Geometry: final body of the model. Coordinates: model frame, mm. Face numbers are marked on the shaded views. A direction names the side the tool comes from. Coordinates: 2 decimals unless noted, no trailing zeros. Write each loop counter-clockwise with the first axis right and the second up, starting at its lowest first coordinate (ties: lowest second). Pieces come first, ordered by that corner, then holes. Notation, with made-up numbers: M 43.25,64 L 80.25,64 A20 cw 80.25,74 Z; hole C 39,74.25 d8. An arc over 180 degrees is marked long. Write item = value, one per line. Start each with the question number.
Item 1: First-contact query: pin 1 Ø3.5 at (x, z) = (5.6, -28.87) entering from +Y; pin 2 Ø0.5 at (x, y) = (7, 3.5) entering from +Z; pin 3 Ø1.6 at (y, z) = (1.5, -35.5) entering from +X. Flat tips, straight axial feed; report the tip coordinate or a pass-through.
Item 2: Section A-A on x = 25.25. Output: boundary loops of the cut face in (y, z), plus the area to 3 significant figures.
Item 3: Pull-direction query (Z, two-part tool) for the marked faces 3 and 4; classes: +Z half, -Z half, draft (parallel to the pull), parting line (faces both ways), or undercut.
Item 4: Reachability of the marked faces 1 and 2 from +Z, -Z, +X, -X, +Y, -Y: full face, straight path, thin tool, end or side. Return the list, or none.
Item 5: Ray query, L1, parallel to X at y = 1.7, z = 2.45; L2, parallel to Z at x = 3, y = 0.35; L3, parallel to Z at x = 16.5, y = 2.75. Return the intervals inside material, ascending. Write a range as [from, to].
Item 6: Section B-B on z = -16. Output: boundary loops of the cut face in (x, y).
Item 7: Section C-C on z = -3. Output: boundary loops of the cut face in (x, y).
from build123d import *

# Parameters (mm, degrees)
SKETCH_1_W           = 20
SKETCH_1_H           = 35.74
EXTRUDE_1_DEPTH      = 4
SKETCH_2_W           = 8.8
SKETCH_2_H           = 8.5
SKETCH_2_H_2         = 9.8
EXTRUDE_2_DEPTH      = 4
SKETCH_3_R           = 13.5
CUT_EXTRUDE_1_DEPTH  = 10
SKETCH_4_W           = 9
SKETCH_4_H           = 5
CUT_EXTRUDE_2_DEPTH  = 1
SKETCH_5_W           = 9.228972975
SKETCH_5_H           = 4
EXTRUDE_3_DEPTH      = 10
SKETCH_6_R           = 1.6
CUT_EXTRUDE_3_DEPTH  = 10
SKETCH_7_R           = 1.6
CUT_EXTRUDE_4_DEPTH  = 55.679901244
SKETCH_8_W           = 11.2
SKETCH_8_H           = 4
EXTRUDE_4_DEPTH      = 4
SKETCH_9_R           = 1.65
CUT_EXTRUDE_5_DEPTH  = 55.679901244
SKETCH_10_W          = 10
SKETCH_10_H          = 4
EXTRUDE_5_DEPTH      = 7
SKETCH_11_R          = 1.65
CUT_EXTRUDE_6_DEPTH  = 8
SKETCH_12_W          = 6.6
SKETCH_12_H          = 5
CUT_EXTRUDE_7_DEPTH  = 1
SKETCH_13_R          = 1.55
CUT_EXTRUDE_8_DEPTH  = 5
SKETCH_14_W          = 18.2
SKETCH_14_H          = 1.73
EXTRUDE_6_DEPTH      = 4
SKETCH_16_W          = 10
SKETCH_16_H          = 8
CUT_EXTRUDE_9_DEPTH  = 1
CUT_EXTRUDE_10_DEPTH = 2.4
FILLET_1_R           = 4
CUT_EXTRUDE_11_DEPTH = 55.679901244
CHAMFER_1_SIZE       = 0.4


with BuildPart() as part:
    # 草图1 → 凸台-拉伸1 (new body)
    with BuildSketch(Plane(origin=(0, 0, 0), x_dir=(1, 0, 0), z_dir=(0, 1, 0))):
        with Locations((10, 17.87)):
            Rectangle(SKETCH_1_W, SKETCH_1_H)
    extrude(amount=EXTRUDE_1_DEPTH)

    # 草图2 → 凸台-拉伸2 (add)
    with BuildSketch(Plane.XZ):
        with Locations((15.6, 4.25)):
            Rectangle(SKETCH_2_W, SKETCH_2_H)
        with Locations((15.6, -40.64)):
            Rectangle(SKETCH_2_W, SKETCH_2_H_2)
    extrude(amount=-EXTRUDE_2_DEPTH)

    # 草图3 → 切除-拉伸1 (cut)
    with BuildSketch(Plane(origin=(0, 0, 0), x_dir=(-1, 0, 0), z_dir=(0, -1, 0))):
        with Locations((-24, 21.6)):
            Circle(SKETCH_3_R)
    extrude(amount=-CUT_EXTRUDE_1_DEPTH, mode=Mode.SUBTRACT)

    # 草图4 → 切除-拉伸2 (cut)
    with BuildSketch(Plane(origin=(0, 0, 0), x_dir=(-1, 0, 0), z_dir=(0, -1, 0))):
        with Locations((-13.5, -0.75)):
            Rectangle(SKETCH_4_W, SKETCH_4_H)
    extrude(amount=-CUT_EXTRUDE_2_DEPTH, mode=Mode.SUBTRACT)

    # 草图5 → 凸台-拉伸3 (add)
    with BuildSketch(Plane(origin=(20, 0, 0), x_dir=(0, 0, -1), z_dir=(1, 0, 0))):
        with Locations((-3.885513513, 2)):
            Rectangle(SKETCH_5_W, SKETCH_5_H)
    extrude(amount=EXTRUDE_3_DEPTH)

    # 草图6 → 切除-拉伸3 (cut)
    with BuildSketch(Plane(origin=(0, 0, 0), x_dir=(-1, 0, 0), z_dir=(0, -1, 0))):
        with Locations(Location((-15.2, 36.59, 0), (0, 0, 90))):
            Circle(SKETCH_6_R)
        with Locations(Location((-25.25, -2.45, 0), (0, 0, 90))):
            Circle(SKETCH_6_R)
    extrude(amount=-CUT_EXTRUDE_3_DEPTH, mode=Mode.SUBTRACT)

    # 草图7 → 切除-拉伸4 (cut, through all)
    with BuildSketch(Plane(origin=(0, 0, 0), x_dir=(-1, 0, 0), z_dir=(0, -1, 0))):
        with Locations(Location((-5.6, 28.87, 0), (0, 0, 90))):
            Circle(SKETCH_7_R)
        with Locations(Location((-5.6, 6.87, 0), (0, 0, 90))):
            Circle(SKETCH_7_R)
    extrude(amount=-CUT_EXTRUDE_4_DEPTH, mode=Mode.SUBTRACT)

    # 草图8 → 凸台-拉伸4 (add)
    with BuildSketch(Plane.XZ):
        with Locations((5.6, -37.74)):
            Rectangle(SKETCH_8_W, SKETCH_8_H)
        with Locations((5.6, 2)):
            Rectangle(SKETCH_8_W, SKETCH_8_H)
    extrude(amount=-EXTRUDE_4_DEPTH)

    # 草图9 → 切除-拉伸5 (cut, through all)
    with BuildSketch(Plane(origin=(0, 0, 0), x_dir=(-1, 0, 0), z_dir=(0, -1, 0))):
        with Locations(Location((-7.6, 35.87, 0), (0, 0, 90))):
            Circle(SKETCH_9_R)
        with Locations((-0.6, -0.13)):
            Circle(SKETCH_9_R)
    extrude(amount=-CUT_EXTRUDE_5_DEPTH, mode=Mode.SUBTRACT)

    # 草图10 → 凸台-拉伸5 (add)
    with BuildSketch(Plane.ZY):
        with Locations((-34.74, 2)):
            Rectangle(SKETCH_10_W, SKETCH_10_H)
        with Locations((-1, 2)):
            Rectangle(SKETCH_10_W, SKETCH_10_H)
    extrude(amount=EXTRUDE_5_DEPTH)

    # 草图11 → 切除-拉伸6 (cut)
    with BuildSketch(Plane(origin=(0, 0, 0), x_dir=(-1, 0, 0), z_dir=(0, -1, 0))):
        with Locations(Location((2.4, 34.87, 0), (0, 0, 90))):
            Circle(SKETCH_11_R)
    extrude(amount=-CUT_EXTRUDE_6_DEPTH, mode=Mode.SUBTRACT)

    # 草图12 → 切除-拉伸7 (cut)
    with BuildSketch(Plane(origin=(0, 0, 0), x_dir=(-1, 0, 0), z_dir=(0, -1, 0))):
        with Locations((-7.9, -0.75)):
            Rectangle(SKETCH_12_W, SKETCH_12_H)
    extrude(amount=-CUT_EXTRUDE_7_DEPTH, mode=Mode.SUBTRACT)

    # 草图13 → 切除-拉伸8 (cut)
    with BuildSketch(Plane(origin=(0, 0, 0), x_dir=(-1, 0, 0), z_dir=(0, -1, 0))):
        with Locations((-0.6, -0.13)):
            Circle(SKETCH_13_R)
    extrude(amount=-CUT_EXTRUDE_8_DEPTH, mode=Mode.SUBTRACT)

    # 草图14 → 凸台-拉伸6 (add)
    with BuildSketch(Plane(origin=(0, 0, 0), x_dir=(-1, 0, 0), z_dir=(0, -1, 0))):
        with Locations((-2.1, -4.865)):
            Rectangle(SKETCH_14_W, SKETCH_14_H)
        with Locations((-2.1, 40.605)):
            Rectangle(SKETCH_14_W, SKETCH_14_H)
    extrude(amount=-EXTRUDE_6_DEPTH)

    # 草图16 → 切除-拉伸9 (cut)
    with BuildSketch(Plane(origin=(0, 4, 0), x_dir=(1, 0, 0), z_dir=(0, 1, 0))):
        with Locations((10.7, 17.87)):
            Rectangle(SKETCH_16_W, SKETCH_16_H)
    extrude(amount=-CUT_EXTRUDE_9_DEPTH, mode=Mode.SUBTRACT)

    # 草图17 → 切除-拉伸10 (cut)
    with BuildSketch(Plane(origin=(0, 0, 0), x_dir=(-1, 0, 0), z_dir=(0, -1, 0))):
        Polygon((-8.833161507, 28.87), (-7.216580754, 26.07), (-3.983419246, 26.07), (-2.366838493, 28.87), (-3.983419246, 31.67), (-7.216580754, 31.67), align=None)
        Polygon((-8.833161507, 6.87), (-7.216580754, 4.07), (-3.983419246, 4.07), (-2.366838493, 6.87), (-3.983419246, 9.67), (-7.216580754, 9.67), align=None)
    extrude(amount=-CUT_EXTRUDE_10_DEPTH, mode=Mode.SUBTRACT)

    # 圆角1
    # the kernel refuses this fillet: 4 mm, written as the material it takes off along each edge
    with BuildSketch(Plane(origin=(11.2, -9.515480808, 8.5), x_dir=(1, 0, 0), z_dir=(0, 1, 0))) as fillet_1_piece_1:
        with BuildLine():
            CenterArc((3.806192323, 4), FILLET_1_R, 197.908633295, 72.091366705)
            Line((0, 2.77), (-0.076123846, 2.7454))
            ThreePointArc((-0.076123846, 2.7454), (-0.08, 1.385), (-0.08, 0))
            Line((-0.08, 0), (0, -0.08))
            Line((0, -0.08), (3.806192323, -0.08))
            Line((3.806192323, -0.08), (3.806192323, 0))
        make_face()
    extrude(amount=23.030961615, mode=Mode.SUBTRACT)
    with BuildSketch(Plane(origin=(11.2, -10, -45.54), x_dir=(0, 0, 1), z_dir=(0, 1, 0))) as fillet_1_piece_2:
        with BuildLine():
            CenterArc((FILLET_1_R, FILLET_1_R), FILLET_1_R, 180, 90)
            Line((0, FILLET_1_R), (-FILLET_1_R * 0.02, FILLET_1_R))
            Line((-FILLET_1_R * 0.02, FILLET_1_R), (-FILLET_1_R * 0.02, -FILLET_1_R * 0.02))
            Line((-FILLET_1_R * 0.02, -FILLET_1_R * 0.02), (FILLET_1_R, -FILLET_1_R * 0.02))
            Line((FILLET_1_R, -FILLET_1_R * 0.02), (FILLET_1_R, 0))
        make_face()
    extrude(amount=24, mode=Mode.SUBTRACT)

    # 草图19 → 切除-拉伸11 (cut, through all)
    with BuildSketch(Plane(origin=(0, 4, 0), x_dir=(1, 0, 0), z_dir=(0, 1, 0))):
        Polygon((0.6, -2.092990915), (2.3, -1.111495458), (2.3, 0.851495458), (0.6, 1.832990915), (-1.1, 0.851495458), (-1.1, -1.111495458), align=None)
        Polygon((-2.4, 32.907009085), (-0.7, 33.888504542), (-0.7, 35.851495458), (-2.4, 36.832990915), (-4.1, 35.851495458), (-4.1, 33.888504542), align=None)
        Polygon((7.6, 33.907009085), (9.3, 34.888504542), (9.3, 36.851495458), (7.6, 37.832990915), (5.9, 36.851495458), (5.9, 34.888504542), align=None)
    extrude(amount=-CUT_EXTRUDE_11_DEPTH, mode=Mode.SUBTRACT)

    # 倒角1
    chamfer_1_edges = [part.edges().sort_by_distance(p)[0] for p in [
        (5.6, 4, -5.27),
        (0, 4, -17.87),
        (-3.5, 4, -29.74),
        (-7, 4, -35.605),
        (22.503096162, 4, 8.5),
        (-3.5, 4, -6),
        (-7, 4, -0.135),
        (2.1, 4, 5.73),
        (11.2, 4, -41.505),
        (2.1, 4, -41.47),
        (13.212093026, 4, -29.716099009),
        (8.101350135, 4, -21.87),
        (5.7, 4, -17.87),
        (9.316079599, 4, -13.87),
        (17.6, 4, -45.54),
        (12.371572875, 4, -44.368427125),
        (12.652471864, 4, 7.734192326),
        (-0.25, 4, 1.602243186),
        (1.45, 4, 1.602243186),
        (2.3, 4, 0.13),
        (1.45, 4, -1.342243186),
        (-0.25, 4, -1.342243186),
        (-1.1, 4, 0.13),
        (-3.25, 4, -33.397756814),
        (-1.55, 4, -33.397756814),
        (-0.7, 4, -34.87),
        (-1.55, 4, -36.342243186),
        (-3.25, 4, -36.342243186),
        (-4.1, 4, -34.87),
        (6.75, 4, -34.397756814),
        (8.45, 4, -34.397756814),
        (9.3, 4, -35.87),
        (8.45, 4, -37.342243186),
        (6.75, 4, -37.342243186),
        (5.9, 4, -35.87),
        (20, 4, -40.016898479),
        (16.035945985, 4, -10.699364989),
        (20, 4, -4.717588008),
        (25, 4, -0.728972975),
        (30, 4, 3.885513513),
        (15.2, 4, -34.99),
        (25.25, 4, 4.05),
        (5.6, 4, -27.27),
    ]]
    chamfer(chamfer_1_edges, length=CHAMFER_1_SIZE)


solid = part.part
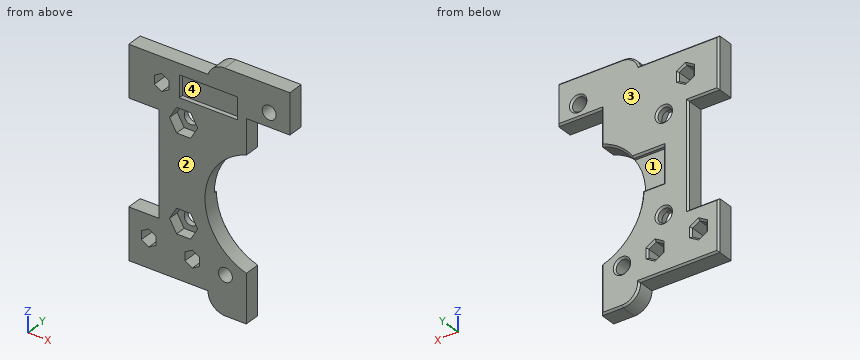
Responses:
q1.pin_1 = 3.75
q1.pin_2 = 5.73
q1.pin_3 = 20
q2.outline = M 0,-0.73 L 3.6,-0.73 L 4,-0.33 L 4,0.45 L 3.6,0.85 L 0,0.85 Z; M 0,4.05 L 3.6,4.05 L 4,4.45 L 4,8.1 L 3.6,8.5 L 0,8.5 Z
q2.area = 23.8 mm²
q3.face_3 = draft
q3.face_4 = undercut
q4.face_1 = +X, +Y
q4.face_2 = +Z, -Z, +X, -X, -Y
q5.L1 = [-7, 23.65], [26.85, 30]
q5.L2 = [-41.47, -29.97], [-27.77, -7.97], [-5.77, 5.73]
q5.L3 = [-45.54, -37.52], [-35.66, -32.82], [-10.38, 8.5]
q6.outline = M 0,0 L 11.72,0 L 11.72,3 L 5.7,3 L 5.7,3.6 L 5.3,4 L 0.4,4 L 0,3.6 Z
q7.outline = M -7,0 L 20,0 L 20,3.6 L 19.6,4 L -6.6,4 L -7,3.6 Z
